from build123d import *

# Parameters (mm, degrees)
EXTRUDE_1_DEPTH = 100
SKETCH_2_R      = 5
EXTRUDE_2_DEPTH = 30


with BuildPart() as part:
    # 草圖1 → 填料-伸長1 (new body)
    with BuildSketch(Plane(origin=(0, 0, 0), x_dir=(1, 0, 0), z_dir=(0, 1, 0))):
        with BuildLine():
            Line((0, 0), (104, 0))
            ThreePointArc((104, 0), (245.421356237, 58.578643763), (304, 200))
            Line((304, 200), (304, 304))
            Line((304, 304), (200, 304))
            ThreePointArc((200, 304), (58.578643763, 245.421356237), (0, 104))
            Line((0, 104), (0, 0))
        make_face()
    extrude(amount=EXTRUDE_1_DEPTH)

    # 草圖2 → 填料-伸長2 (add)
    with BuildSketch(Plane(origin=(0, 100, 0), x_dir=(1, 0, 0), z_dir=(0, 1, 0))):
        with Locations(Location((15, 15, 0), (0, 0, 90))):
            Circle(SKETCH_2_R)
        with Locations(Location((289, 289, 0), (0, 0, 90))):
            Circle(SKETCH_2_R)
    extrude(amount=EXTRUDE_2_DEPTH)


solid = part.part
Input: part model. Units: mm. Frame: model coordinates. A direction names the side the tool comes from. Coordinates: 2 decimals unless noted, no trailing zeros. Loops run counter-clockwise (first coordinate to the right, second up) from the corner with the lowest first, then second, coordinate; pieces in that order, holes last.
Q1. Contact query for flat-ended pins moving along their axis: pin 1 (10 mm diameter, centred on y = 19.5, z = -196, fed in from -X); pin 2 (10 mm diameter, centred on x = 185.5, y = 21, fed in from +Z); pin 3 (5 mm diameter, centred on x = 177.5, z = -209.5, fed in from +Y). Output: stop coordinate, or through.
Q2. Cut plane A-A (y = 117.5). Output: boundary loops of the cut face in (x, z).
Q3. Set-up query: faces 1 (the face through (285, 115, -292)), 2 (the face through (243.858, 49.3, -57.032)). Return all of +Z, -Z, +X, -X, +Y, -Y with unobstructed straight access to the full face (end or side cutting, diameter ignored); none if empty.
Q4. Material intervals for line 1 (Y direction, x = 227, z = -236.5); line 2 (Z direction, x = 45.5, y = 98); line 3 (X direction, y = 43, z = -228.5), sorted ascending.
Q5. Cut plane D-D (y = 84). Output: boundary loops of the cut face in (x, z), then the cut area to 3 significant figures.
Q6. Cut plane B-B (z = -289). Output: boundary loops of the cut face in (x, y), then the cut area to 3 significant figures.
Q7. Cut plane C-C (x = 15). Output: boundary loops of the cut face in (y, z).
Working result:
1. pin 1: stops at x = 19.91
1. pin 2: stops at z = -15.21
1. pin 3: stops at y = 100
2. outline: circle Ø10 at (15, -15); circle Ø10 at (289, -289)
3. face 1: +Y
3. face 2: +Z, +X, +Y, -Y
4. line 1: y = 0 to 100
4. line 2: z = -231 to 0
4. line 3: x = 43.48 to 304
5. outline: (0, -104) arc R200 ccw to (200, -304) - (304, -304) - (304, -200) arc R200 ccw to (104, 0) - (0, 0) - close
5. area: 75,200 mm2
6. outline: (124.01, 0) - (304, 0) - (304, 100) - (294, 100) - (294, 130) - (284, 130) - (284, 100) - (124.01, 100) - close
6. area: 18,300 mm2
7. outline: (0, -179.99) - (100, -179.99) - (100, -20) - (130, -20) - (130, -10) - (100, -10) - (100, 0) - (0, 0) - close
